Model file for the job. Use its own axes, mm. Coordinates: 2 decimals unless noted, no trailing zeros. Write each loop counter-clockwise with the first axis right and the second up, starting at its lowest first coordinate (ties: lowest second). Pieces come first, ordered by that corner, then holes. Notation, with made-up numbers: M 67,-5.5 L 90,-5.5 A20 cw 90,27.5 Z; hole C 49.25,49 d11. An arc over 180 degrees is marked long. Put each result on its own line as item: value. Start each with the question number.
Q1. Cut at A-A (y = 42.5). Write the cut outline in (x, z).
Q2. Cut at C-C (z = 10.5). Write the cut outline in (x, y).
Q3. Cut at B-B (x = -255.5). Write the cut outline in (y, z).
Q4. Pull direction Y, two halves, no side cores. Call faces 1 (the flat face through (-246, 48, -15)), 2 (the cylindrical face through (-232.96, 41.87, -0.21)), 3 (the cylindrical face through (-257.44, 38.21, 0.21)): pulls with the +Y half, pulls with the -Y half, needs draft (parallel to the pull), parting line crosses it, or undercut.
Q5. Drill centre lines: line 1 along Y through (x, z) = (-255, 0.5) (3 decimals); line 2 along X through (y, z) = (41, -7.5); line 3 along X through (y, z) = (42.75, 10.75). Where is each one in solid material? Low to high.
Q6. Cut at D-D (y = 56.5). Write the cut outline in (x, z), then the cut area to 3 significant figures.
Q7. Drop flat-ended pins along their axis: pin 1 (4 mm diameter, centred on x = -230.5, z = 2.5, fed in from -Y); pin 2 (10 mm diameter, centred on y = 49.5, z = -11.5, fed in from +X); pin 3 (6 mm diameter, centred on y = 45, z = 0, fed in from +X). Give the stop position or say it passes through.
```python
from build123d import *

# Parameters (mm, degrees)
SKETCH1_R                = 2
BOSS_EXTRUDE1_DEPTH      = 15
BOSS_EXTRUDE1_DEPTH_BACK = 15


with BuildPart() as part:
    # Sketch1 → Boss-Extrude1 (new body, two sides)
    with BuildSketch(Plane.XY) as boss_extrude1_sk:
        with BuildLine():
            Line((-250.73011668, 64.896080811), (-227.748783387, 45.61245252))
            ThreePointArc((-227.748783387, 45.61245252), (-226.264258331, 40.072129588), (-230.962721435, 36.782230305))
            Line((-230.962721435, 36.782230305), (-253.944054729, 36.782230305))
            ThreePointArc((-253.944054729, 36.782230305), (-257.479588635, 38.246696399), (-258.944054729, 41.782230305))
            Line((-258.944054729, 41.782230305), (-258.944054729, 61.065858595))
            ThreePointArc((-258.944054729, 61.065858595), (-256.057146037, 65.597397531), (-250.73011668, 64.896080811))
        make_face()
        with Locations((-253.944054729, 61.065858595)):
            Circle(SKETCH1_R, mode=Mode.SUBTRACT)
        with Locations((-230.962721435, 41.782230305)):
            Circle(SKETCH1_R, mode=Mode.SUBTRACT)
    extrude(amount=BOSS_EXTRUDE1_DEPTH)
    extrude(boss_extrude1_sk.sketch, amount=-BOSS_EXTRUDE1_DEPTH_BACK)


solid = part.part
```
Computed values:
1. outline: M -258.94,-15 L -232.83,-15 L -232.83,15 L -258.94,15 Z; M -229.1,-15 L -226.01,-15 L -226.01,15 L -229.1,15 Z
2. outline: M -258.94,41.78 A5 ccw -253.94,36.78 L -230.96,36.78 A5 ccw -227.75,45.61 L -250.73,64.9 A5 ccw -258.94,61.07 Z; hole C -253.94,61.07 d4; hole C -230.96,41.78 d4
3. outline: M 37.03,-15 L 59.81,-15 L 59.81,15 L 37.03,15 Z; M 62.32,-15 L 65.82,-15 L 65.82,15 L 62.32,15 Z
4. face 1: needs draft
4. face 2: undercut
4. face 3: pulls with the -Y half
5. line 1: 36.895 to 59.367, 62.764 to 65.953
5. line 2: -258.88 to -232.8, -229.12 to -226.02
5. line 3: -258.94 to -232.71, -229.21 to -226.06
6. outline: M -258.94,-15 L -240.72,-15 L -240.72,15 L -258.94,15 Z
6. area: 547 mm2
7. pin 1: y = 36.78
7. pin 2: x = -226.77
7. pin 3: x = -225.97
